```python
from build123d import *

# Parameters (mm, degrees)
SKETCH1_R                   = 31.75
BOSS_EXTRUDE1_DEPTH         = 6.35
SKETCH2_R                   = 6.35
BOSS_EXTRUDE2_DEPTH         = 6.35
SKETCH3_R                   = 2.3749
CUT_EXTRUDE1_DEPTH          = 47.6627796
F_3_8_16_TAPPED_HOLE1_D     = 7.9375
F_3_8_16_TAPPED_HOLE1_DEPTH = 26.924
F_3_8_16_TAPPED_HOLE1_TIP   = 2.384665582


with BuildPart() as part:
    # Sketch1 → Boss-Extrude1 (new body)
    with BuildSketch(Plane(origin=(0, 0, 0), x_dir=(1, 0, 0), z_dir=(0, 1, 0))):
        with Locations(Location((0, 0, 0), (0, 0, 270))):
            Circle(SKETCH1_R)
    extrude(amount=BOSS_EXTRUDE1_DEPTH)

    # Sketch2 → Boss-Extrude2 (add)
    with BuildSketch(Plane(origin=(0, 6.35, 0), x_dir=(1, 0, 0), z_dir=(0, 1, 0))):
        with Locations(Location((0, 0, 0), (0, 0, 270))):
            Circle(SKETCH2_R)
    extrude(amount=BOSS_EXTRUDE2_DEPTH)

    # Sketch3 → Cut-Extrude1 (cut, through all)
    with BuildSketch(Plane(origin=(0, 12.7, 0), x_dir=(1, 0, 0), z_dir=(0, 1, 0))):
        with Locations(Location((0, 0, 0), (0, 0, 270))):
            Circle(SKETCH3_R)
    extrude(amount=-CUT_EXTRUDE1_DEPTH, mode=Mode.SUBTRACT)

    # 3/8-16 Tapped Hole1
    with Locations(Plane(origin=(0, 6.35, 0), x_dir=(1, 0, 0), z_dir=(0, 1, 0))):
        with Locations((0, 19.05), (19.05, 0), (0, -19.05), (-19.05, 0)):
            Hole(F_3_8_16_TAPPED_HOLE1_D / 2, depth=F_3_8_16_TAPPED_HOLE1_DEPTH)
            with Locations((0, 0, -(F_3_8_16_TAPPED_HOLE1_DEPTH + F_3_8_16_TAPPED_HOLE1_TIP / 2))):  # 118° drill point
                Cone(0, F_3_8_16_TAPPED_HOLE1_D / 2, F_3_8_16_TAPPED_HOLE1_TIP, mode=Mode.SUBTRACT)


solid = part.part
```
Could you check a few things on this model? Use its own coordinates, in mm. Coordinates: 2 decimals unless noted, no trailing zeros. Loops run counter-clockwise (first coordinate to the right, second up) from the corner with the lowest first, then second, coordinate; pieces in that order, holes last. Notation, with made-up numbers: M 72.5,-35 L 94.5,-35 A21 cw 94.5,-7 Z; hole C -12.75,-2 d3. An arc over 180 degrees is marked long. Put each result on its own line as item: value. Start each with the question number.
(1) Suppose I cut it at A-A on x = -19.05. Please give me the cut outline in (y, z), then the cut area to 3 significant figures.
(2) Will these pins go through, and if not, where does the flat tip stop? P1, Ø12.5, axis at x = 0, z = -19.05, coming from the +Y side; P2, Ø5, axis at x = -19.05, z = 0, coming from the -Y side; P3, Ø6, axis at x = -24.5, y = 7, coming from the +Z side; P4, Ø1.5, axis at x = 7.5, y = 2, coming from the -Z side.
(3) Suppose I cut it at C-C on x = 0. Please give me the cut outline in (y, z).
(4) Suppose I cut it at B-B on z = 0. Please give me the cut outline in (x, y).
(5) I need wall thicknesses on line 1 (Z direction, x = -2.5, y = 3.25); line 2 (Z direction, x = 3, y = 3.5); line 3 (X direction, y = 4.75, z = -1.5). Which ranges of each line are inside material? Lowest first, please. Write a range as from..to.
(6) Suppose I cut it at D-D on z = 19.05. Please give me the cut outline in (x, y), then the cut area to 3 significant figures.
(7) Thinking about a two-plate mould opening in Z: for faces 1 (the face through (0.713, 6.439, 2.265)), 2 (the face through (-3.86, 9.48, -5.04)), 3 (the face through (0, 12.7, 3)), which applies, pulls with the +Z half, pulls with the -Z half, needs draft (parallel to the pull), parting line crosses it, or undercut?
Solutions:
1. outline: M 0,-25.4 L 6.35,-25.4 L 6.35,-3.97 L 0,-3.97 Z; M 0,3.97 L 6.35,3.97 L 6.35,25.4 L 0,25.4 Z
1. area: 272 mm2
2. P1: stops at y = 6.35
2. P2: passes through
2. P3: stops at z = 23.3
2. P4: stops at z = -31.02
3. outline: M 0,-31.75 L 6.35,-31.75 L 6.35,-23.02 L 0,-23.02 Z; M 0,-15.08 L 6.35,-15.08 L 6.35,-6.35 L 12.7,-6.35 L 12.7,-2.37 L 0,-2.37 Z; M 0,2.37 L 12.7,2.37 L 12.7,6.35 L 6.35,6.35 L 6.35,15.08 L 0,15.08 Z; M 0,23.02 L 6.35,23.02 L 6.35,31.75 L 0,31.75 Z
4. outline: M -31.75,0 L -23.02,0 L -23.02,6.35 L -31.75,6.35 Z; M -15.08,0 L -2.37,0 L -2.37,12.7 L -6.35,12.7 L -6.35,6.35 L -15.08,6.35 Z; M 2.37,0 L 15.08,0 L 15.08,6.35 L 6.35,6.35 L 6.35,12.7 L 2.37,12.7 Z; M 23.02,0 L 31.75,0 L 31.75,6.35 L 23.02,6.35 Z
5. line 1: z = -31.65..-22.13, -15.97..15.97, 22.13..31.65
5. line 2: z = -31.61..-21.65, -16.45..16.45, 21.65..31.61
5. line 3: x = -31.71..-22.72, -15.38..-1.84, 1.84..15.38, 22.72..31.71
6. outline: M -25.4,0 L -3.97,0 L -3.97,6.35 L -25.4,6.35 Z; M 3.97,0 L 25.4,0 L 25.4,6.35 L 3.97,6.35 Z
6. area: 272 mm2
7. face 1: undercut
7. face 2: parting line crosses it
7. face 3: needs draft
